```python
from build123d import *

# Parameters (mm, degrees)
F0_R     = 30
F0_W     = 44
F0_H     = 39
F1_DEPTH = 7
F2_SIZE  = 3


with BuildPart() as f1:
    # F0 (on Top) → F1 (new body)
    with BuildSketch(Plane.XY):
        Circle(F0_R)
        Rectangle(F0_W, F0_H, mode=Mode.SUBTRACT)
    extrude(amount=F1_DEPTH)

    # F2
    f2_edges = [f1.edges().sort_by_distance(p)[0] for p in [
        (-22, 19.5, 3.5),
        (22, 19.5, 3.5),
        (-22, -19.5, 3.5),
        (22, -19.5, 3.5),
    ]]
    chamfer(f2_edges, length=F2_SIZE)


solid = f1.part
```
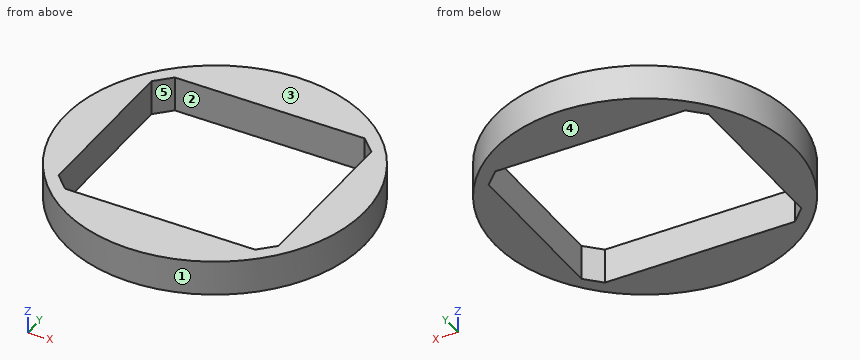
Geometry: final body of the model. Coordinates: model frame, mm. Face numbers are marked on the shaded views. A direction names the side the tool comes from. Coordinates: 2 decimals unless noted, no trailing zeros. Order: outer loops, then holes, each group sorted by start corner. A loop starts at its lowest first (then second) coordinate and runs counter-clockwise, first axis right, second up.
Item 1: Section query B-B (x = 0). Output: boundary loops of the cut face in (y, z).
Answer:
outline: (-30, 0) - (-19.5, 0) - (-19.5, 7) - (-30, 7) - close; (19.5, 0) - (30, 0) - (30, 7) - (19.5, 7) - close
Item 2: Material intervals for line 1 along Y through (x, z) = (8.5, 5.5); line 2 along Y through (x, z) = (-18, 4.75); line 3 along X through (y, z) = (-7.5, 1.25), sorted ascending.
Answer:
line 1: y = -28.77 to -19.5, 19.5 to 28.77
line 2: y = -24 to -19.5, 19.5 to 24
line 3: x = -29.05 to -22, 22 to 29.05
Item 3: Section query C-C (z = 1.25). Output: boundary loops of the cut face in (x, y).
Answer:
outline: circle Ø60 at (0, 0); hole (-22, -16.5) - (-19, -19.5) - (19, -19.5) - (22, -16.5) - (22, 16.5) - (19, 19.5) - (-19, 19.5) - (-22, 16.5) - close
Item 4: Section query A-A (y = 0). Output: boundary loops of the cut face in (x, z).
Answer:
outline: (-30, 0) - (-22, 0) - (-22, 7) - (-30, 7) - close; (22, 0) - (30, 0) - (30, 7) - (22, 7) - close
Item 5: Access query for the marked faces 4 and 5. Directions: +Z, -Z, +X, -X, +Y, -Y. A direction counts if a zero-diameter tool reaches every point of the face in a straight line with its end or side. Return the directions, or none.
Answer:
face 4: -Z, +X, -X, +Y, -Y
face 5: +Z, -Z
Item 6: Contact query for flat-ended pins moving along their axis: P1, Ø2, axis at x = -7.5, z = 4, coming from the -Y side; P2, Ø4, axis at y = 6, z = 2, coming from the +X side. Output: stop coordinate, or through.
Answer:
P1: stops at y = -29.29
P2: stops at x = 29.73
Item 7: Draft query along Y for the marked faces 1, 2 and 3. Return one class per face: released by +Y, released by -Y, zero draft, split by the parting line, or undercut.
Answer:
face 1: split by the parting line
face 2: undercut
face 3: zero draft
